Work out the finished part from the listing and answer in its coordinate system (mm). A direction names the side the tool comes from. Give positions to 0.01 mm unless a question says otherwise; leave off trailing zeros. Write each loop counter-clockwise with the first axis right and the second up, starting at its lowest first coordinate (ties: lowest second). Pieces come first, ordered by that corner, then holes.
1) A tool of negligible diameter and unlimited length cuts with its end or side. For faces 1 (the face through (-33.5, -113, 59)), 2 (the face through (-15, -92, 66)), 3 (the face through (-8.5, -92, 75)), 4 (the face through (-5.5, -88, 70)), 5 (the face through (-30, -90, 58)), from which of +Z, -Z, +X, -X, +Y, -Y can it reach the whole face along a straight path? Write none if from no direction.
2) Find section A-A (x = -13.5). Determine the outline of the cut face in (y, z), plus the area to 3 significant figures.
3) Straight lines are drawn through the part: probe 1 along X at (y, z) = (-110.5, 54.4); probe 2 along X at (y, z) = (-92, 63.5); probe 3 along Z at (x, y) = (3.5, -91.25). For each, find the intervals that lie inside material, in ascending order.
4) Find section D-D (y = -94). Determine the outline of the cut face in (x, z).
5) Find section C-C (z = 70.5). Determine the outline of the cut face in (x, y).
6) Determine the mould class of faces 6 (the face through (-10, -92, 67)), 7 (the face through (-35.84, -96.68, 59.48)), 8 (the face through (-33.15, -94.93, 55.46)), 9 (the face through (-13.695, -109.013, 54.972)) for opening direction Y: pulls with the +Y half, pulls with the -Y half, needs draft (parallel to the pull), parting line crosses it, or undercut.
7) Given pin 1 Ø6 at (x, y) = (-11, -108) entering from +Z; pin 2 Ø3 at (x, y) = (-36, -103.5) entering from +Z; pin 3 Ø1 at (x, z) = (-10, 65.5) entering from -Y; pin 4 Ø12 at (x, z) = (-17, 77.5) entering from +Y, each flat-ended and moving along its own axis, determine where each tip first touches the part or whether it passes through.
8) Find section B-B (y = -110.5). Determine the outline of the cut face in (x, z).
```python
from build123d import *

# Parameters (mm, degrees)
CYLINDER015_W               = 7.75
CYLINDER015_H               = 10
CYLINDER015_ANGLE           = 90
CYLINDER014_R               = 5.75
CYLINDER014_DEPTH           = 10
CYLINDER014_PLACEMENT_ANGLE = 285
CYLINDER013_R               = 3
CYLINDER013_DEPTH           = 10
CYLINDER_R                  = 2.8
CYLINDER_DEPTH              = 19
BOX_W                       = 25
BOX_H                       = 10
BOX_DEPTH                   = 16
CYLINDER011_R               = 2
CYLINDER011_DEPTH           = 20
CYLINDER012_R               = 1.5
CYLINDER012_DEPTH           = 42
BOX020_W                    = 18
BOX020_H                    = 50
BOX020_DEPTH                = 40
BOX021_W                    = 9
BOX021_H                    = 32
BOX021_DEPTH                = 3
BOX018_W                    = 8
BOX018_H                    = 42
BOX018_DEPTH                = 48
BOX019_W                    = 10
BOX019_H                    = 10
BOX019_DEPTH                = 10
CUT_PLACEMENT_ANGLE         = 180
BOX022_W                    = 30
BOX022_H                    = 10
BOX022_DEPTH                = 19


with BuildPart() as cylinder015:
    # Cylinder015 → Cylinder015 (revolve)
    with BuildSketch(Plane(origin=(-32.5, -92, 58), x_dir=(0, 1, 0), z_dir=(1, 0, 0))):
        with Locations((3.875, 5)):
            Rectangle(CYLINDER015_W, CYLINDER015_H)
    revolve(axis=Axis((-32.5, -92, 58), (0, 0, 1)), revolution_arc=CYLINDER015_ANGLE)


with BuildPart() as cylinder014:
    # Cylinder014 → Cylinder014 (new body)
    with BuildSketch(Plane.XY):
        Circle(CYLINDER014_R)
    extrude(amount=CYLINDER014_DEPTH)


with BuildPart() as cylinder014_1:
    # Cylinder014 placement: moved
    add(cylinder014.part.moved(Location((-32.5, -92, 58))).rotate(Axis((-32.5, -92, 58), (0, 0, 1)), CYLINDER014_PLACEMENT_ANGLE))


with BuildPart() as cylinder013:
    # Cylinder013 → Cylinder013 (new body)
    with BuildSketch(Plane(origin=(-32.5, -92, 53), x_dir=(1, 0, 0), z_dir=(0, 0, 1))):
        Circle(CYLINDER013_R)
    extrude(amount=CYLINDER013_DEPTH)


with BuildPart() as cylinder:
    # Cylinder → Cylinder (new body)
    with BuildSketch(Plane(origin=(3.5, -80, 70.5), x_dir=(1, 0, 0), z_dir=(0, -1, 0))):
        Circle(CYLINDER_R)
    extrude(amount=CYLINDER_DEPTH)


with BuildPart() as fusion002:
    # Box → Box (new body)
    with BuildSketch(Plane(origin=(10.5, -90, 58), x_dir=(0, 0, 1), z_dir=(-1, 0, 0))):
        with Locations((12.5, 5)):
            Rectangle(BOX_W, BOX_H)
    extrude(amount=BOX_DEPTH)

    # Fusion002: union Cylinder
    add(cylinder.part)


with BuildPart() as cylinder001:
    # Cylinder011 → Cylinder011 (new body)
    with BuildSketch(Plane(origin=(13.5, 87, 63.5), x_dir=(-1, 0, 0), z_dir=(0, 1, 0))):
        Circle(CYLINDER011_R)
    extrude(amount=CYLINDER011_DEPTH)


with BuildPart() as cut001:
    # Cylinder012 → Cylinder012 (new body)
    with BuildSketch(Plane(origin=(13.5, 110.5, 42.5), x_dir=(-1, 0, 0), z_dir=(0, 0, 1))):
        Circle(CYLINDER012_R)
    extrude(amount=CYLINDER012_DEPTH)


with BuildPart() as gpscut:
    # Box020 → Box020 (new body)
    with BuildSketch(Plane(origin=(33.5, 97, 57), x_dir=(0, 0, 1), z_dir=(-1, 0, 0))):
        with Locations((9, 25)):
            Rectangle(BOX020_W, BOX020_H)
    extrude(amount=BOX020_DEPTH)


with BuildPart() as fusion001:
    # Box021 → Box021 (new body)
    with BuildSketch(Plane(origin=(15, 87, 63), x_dir=(0, 0, 1), z_dir=(-1, 0, 0))):
        with Locations((4.5, 16)):
            Rectangle(BOX021_W, BOX021_H)
    extrude(amount=BOX021_DEPTH)

    # Fusion001: union Cylinder001, cut001, gpsCut
    add(cylinder001.part)
    add(cut001.part)
    add(gpscut.part)


with BuildPart() as shell:
    # Box018 → Box018 (new body)
    with BuildSketch(Plane(origin=(37.5, 87, 53), x_dir=(0, 0, 1), z_dir=(-1, 0, 0))):
        with Locations((4, 21)):
            Rectangle(BOX018_W, BOX018_H)
    extrude(amount=BOX018_DEPTH)


with BuildPart() as obj1:
    # Box019 → Box019 (new body)
    with BuildSketch(Plane(origin=(18.5, 87, 57), x_dir=(0, 0, 1), z_dir=(-1, 0, 0))):
        with Locations((5, 5)):
            Rectangle(BOX019_W, BOX019_H)
    extrude(amount=BOX019_DEPTH)

    # Fusion: union shell
    add(shell.part)

    # Cut: cut Fusion001
    add(fusion001.part, mode=Mode.SUBTRACT)


with BuildPart() as obj1_1:
    # Cut placement: moved
    add(obj1.part.rotate(Axis((0, 0, 0), (0, 0, 1)), CUT_PLACEMENT_ANGLE))


with BuildPart() as gpsholder002:
    # Box022 → Box022 (new body)
    with BuildSketch(Plane(origin=(10.5, -97, 53), x_dir=(0, 0, 1), z_dir=(-1, 0, 0))):
        with Locations((15, 5)):
            Rectangle(BOX022_W, BOX022_H)
    extrude(amount=BOX022_DEPTH)

    # Fusion003: union obj1
    add(obj1_1.part)

    # Cut001: cut Fusion002
    add(fusion002.part, mode=Mode.SUBTRACT)

    # Cut002: cut Cylinder013
    add(cylinder013.part, mode=Mode.SUBTRACT)

    # Cut003: cut Cylinder014
    add(cylinder014_1.part, mode=Mode.SUBTRACT)

    # Cut004: cut Cylinder015
    add(cylinder015.part, mode=Mode.SUBTRACT)


solid = gpsholder002.part
```
Results:
1. face 1: +Z, -Y
1. face 2: +Z, +Y, -Y
1. face 3: +Z, -X, +Y, -Y
1. face 4: +Z, +X, +Y
1. face 5: +Z
2. outline: (-129, 53) - (-112, 53) - (-112, 57) - (-129, 57) - close; (-109, 53) - (-87, 53) - (-87, 61.5) - (-97, 61.5) - (-97, 57) - (-109, 57) - close
2. area: 201 mm2
3. probe 1: x = -37.5 to -15, -12 to 10.5
3. probe 2: x = -18.5 to -15.5, -11.5 to 10.5
3. probe 3: z = 53 to 67.7, 73.3 to 83
4. outline: (-37.5, 53) - (-34.74, 53) - (-34.74, 58) - (-37.5, 58) - close; (-30.26, 53) - (10.5, 53) - (10.5, 83) - (-8.5, 83) - (-8.5, 67) - (-12, 67) - (-12, 64.82) arc R2 cw (long way) to (-15, 64.82) - (-15, 67) - (-18.5, 67) - (-18.5, 61) - (-27.11, 61) - (-27.11, 58) - (-30.26, 58) - close; hole circle Ø5.6 at (3.5, 70.5)
5. outline: (-8.5, -97) - (0.7, -97) - (0.7, -90) - (-5.5, -90) - (-5.5, -87) - (-8.5, -87) - close; (6.3, -97) - (10.5, -97) - (10.5, -90) - (6.3, -90) - close
6. face 6: needs draft
6. face 7: pulls with the +Y half
6. face 8: undercut
6. face 9: undercut
7. pin 1: stops at z = 57
7. pin 2: stops at z = 61
7. pin 3: stops at y = -97
7. pin 4: passes through
8. outline: (-37.5, 53) - (-15, 53) - (-15, 57) - (-33.5, 57) - (-33.5, 61) - (-37.5, 61) - close; (-12, 53) - (10.5, 53) - (10.5, 61) - (6.5, 61) - (6.5, 57) - (-12, 57) - close
